Work out the finished part from the listing and answer in its coordinate system (mm). Face numbers are marked on the shaded views. A direction names the side the tool comes from. Give positions to 0.01 mm unless a question says otherwise; leave off trailing zeros. Loops run counter-clockwise (first coordinate to the right, second up) from the corner with the lowest first, then second, coordinate; pieces in that order, holes last. Notation, with made-up numbers: (5, -9.75) - (19, -9.75) arc R27 ccw to (19, 14.25) - close; hole circle Ø5 at (22, -15.75). An arc over 180 degrees is marked (long way). One line per item, written item: value.
from build123d import *

# Parameters (mm, degrees)
SKETCH1_W           = 39.466666666
SKETCH1_H           = 16
SKETCH1_R           = 1.866666667
BOSS_EXTRUDE1_DEPTH = 6


with BuildPart() as part:
    # Sketch1 → Boss-Extrude1 (new body)
    with BuildSketch(Plane(origin=(0, 0, 0), x_dir=(0, -1, 0), z_dir=(1, 0, 0))):
        with Locations((0.004714435, 11.349547327)):
            Rectangle(SKETCH1_W, SKETCH1_H)
        with Locations(Location((16, 10.666666667, 0), (0, 0, 90))):
            Circle(SKETCH1_R, mode=Mode.SUBTRACT)
        with Locations(Location((-16, 10.666666667, 0), (0, 0, 90))):
            Circle(SKETCH1_R, mode=Mode.SUBTRACT)
        Polygon((-3.417883139, 17.373319057), (-6.923323696, 11.397376747), (-3.500726123, 5.373605017), (3.427312009, 5.325775598), (6.932752566, 11.301717908), (3.510154993, 17.325489638), align=None, mode=Mode.SUBTRACT)
    extrude(amount=BOSS_EXTRUDE1_DEPTH)


solid = part.part
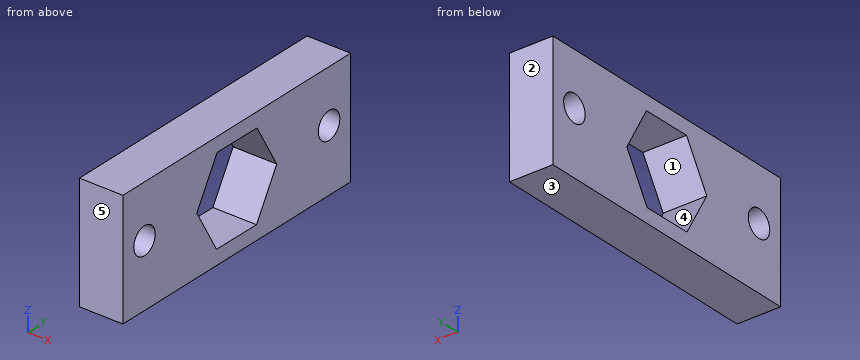
1. Section D-D (z = -6.5) is taken. Write down the section's boundary in (x, y), and give its area (3 significant figures).
Output:
outline: (0, -19.74) - (6, -19.74) - (6, -4.12) - (0, -4.12) - close; (0, 4.14) - (6, 4.14) - (6, 19.73) - (0, 19.73) - close
area: 187 mm²
2. For the marked faces 1 and 2, determine the directions among +Z, -Z, +X, -X, +Y, -Y from which every point of the face is accessible in a straight line to the end or side of a thin tool.
Output:
face 1: +X, -X
face 2: +Z, -Z, +X, -X, +Y
3. The mould has two halves that part along Z. Classify the marked faces 3, 4 and 5: released by +Z, released by -Z, zero draft, split by the parting line, or undercut.
Output:
face 3: released by -Z
face 4: undercut
face 5: zero draft
4. Find the intervals of material crossed by line 1 along Y through (x, z) = (1.5, -9.25); line 2 along Y through (x, z) = (0.65, -10.75); line 3 along Y through (x, z) = (4.95, -7.5), in increasing order.
Output:
line 1: y = -19.74 to -17.22, -14.78 to -5.73, 5.7 to 14.78, 17.22 to 19.73
line 2: y = -19.74 to -17.86, -14.14 to -6.61, 6.56 to 14.14, 17.86 to 19.73
line 3: y = -19.74 to -4.7, 4.71 to 19.73
5. Flat-ended cylindrical pins translate along their axes: pin 1 Ø2 at (y, z) = (16, -10.67) entering from +X; pin 2 Ø6 at (y, z) = (-16, -10.67) entering from -X. Find the tip coordinate at first contact, or state that the pin passes through.
Output:
pin 1: passes through
pin 2: stops at x = 0
6. Section C-C (z = -11.75) is taken. Write down the section's boundary in (x, y).
Output:
outline: (0, -19.74) - (6, -19.74) - (6, -17.52) - (0, -17.52) - close; (0, -14.48) - (6, -14.48) - (6, -6.68) - (0, -6.68) - close; (0, 6.72) - (6, 6.72) - (6, 14.48) - (0, 14.48) - close; (0, 17.52) - (6, 17.52) - (6, 19.73) - (0, 19.73) - close
7. Section A-A (y = 16) is taken. Write down the section's boundary in (x, z).
Output:
outline: (0, -19.35) - (6, -19.35) - (6, -12.53) - (0, -12.53) - close; (0, -8.8) - (6, -8.8) - (6, -3.35) - (0, -3.35) - close
8. Section B-B (x = 4.25) is taken. Write down the section's boundary in (y, z).
Output:
outline: (-19.74, -19.35) - (19.73, -19.35) - (19.73, -3.35) - (-19.74, -3.35) - close; hole circle Ø3.73 at (-16, -10.67); hole (-6.93, -11.3) - (-3.51, -17.33) - (3.42, -17.37) - (6.92, -11.4) - (3.5, -5.37) - (-3.43, -5.33) - close; hole circle Ø3.73 at (16, -10.67)
